Verification items for the finished model (mm, model axes). A direction names the side the tool comes from. Coordinates: 2 decimals unless noted, no trailing zeros. Order: outer loops, then holes, each group sorted by start corner. A loop starts at its lowest first (then second) coordinate and runs counter-clockwise, first axis right, second up. Notation, with made-up numbers: (-14.5, 8) -> (4.5, 8) arc R15 ccw to (4.5, 27) -> close; hole circle Ø5 at (45.25, -14). An arc over 180 degrees is marked (long way). Use CSV: the item, a comma, the result in double quotes. Start each with the question number.
1) Scan lines: line 1 along Z through (x, y) = (-4.25, -8); line 2 along X through (y, z) = (-0.5, 37); line 3 along X through (y, z) = (-4.25, 6.5). Record each from-to range of solid material in increasing order.
2) Sectioned sample at B-B on z = 7. Record the boundary of the cut face in (x, y).
3) Sectioned sample at D-D on y = 8.5. Record the boundary of the cut face in (x, z).
4) Tool access check on faces 1 (the flat face through (0, 7, 55)), 2 (the cylindrical face through (9.237, -3.83, 27.115)). Record the directions out of +Z, -Z, +X, -X, +Y, -Y that give a thin tool (end or side, any length) a straight path to the whole face; none if there is none.
5) Sectioned sample at A-A on y = -5.75. Record the boundary of the cut face in (x, z).
6) Go/stop test with flat-tipped pins: pin 1 (1 mm diameter, centred on x = -1.5, z = 12, fed in from -Y); pin 2 (6 mm diameter, centred on x = -6, z = 38.5, fed in from +Y); pin 3 (6 mm diameter, centred on x = -7, z = 16.5, fed in from -Y). Record where each tip stops, or that it passes through.
7) Sectioned sample at C-C on y = 3. Record the boundary of the cut face in (x, z), then the cut area to 3 significant figures.
8) Release check for a two-part mould opening along Y. For faces 3 (the flat face through (0, 5, 57)), 4 (the cylindrical face through (-0.14, 0.18, 3.29)), 5 (the flat face through (0, 0, 0)), 6 (the cylindrical face through (0, -7, 57)) record: released by +Y, released by -Y, zero draft, split by the parting line, or undercut.
from build123d import *

# Parameters (mm, degrees)
ESBO_O1_R                         = 10
RESSALTO_EXTRUS_O1_DEPTH          = 60
CORTE_EXTRUS_O1_START             = -5
ESBO_O7_R                         = 10
ESBO_O7_R_2                       = 7
CORTE_EXTRUS_O1_DEPTH             = 5
CORTE_EXTRUS_O2_START             = -5
CORTE_EXTRUS_O2_DEPTH             = 5
FURO_COM_FOLGA_DE_M21_D           = 2.6
FURO_COM_FOLGA_DE_M21_CSINK_D     = 2.65
FURO_COM_FOLGA_DE_M21_CSINK_ANGLE = 90


with BuildPart() as part:
    # Esboço1 → Ressalto-extrusão1 (new body)
    with BuildSketch(Plane.XY):
        Circle(ESBO_O1_R)
    extrude(amount=RESSALTO_EXTRUS_O1_DEPTH)

    # Esboço7 → Corte-extrusão1 (cut)
    with BuildSketch(Plane.XY.offset(60).offset(CORTE_EXTRUS_O1_START)):
        Circle(ESBO_O7_R)
        Circle(ESBO_O7_R_2, mode=Mode.SUBTRACT)
    extrude(amount=CORTE_EXTRUS_O1_DEPTH, mode=Mode.SUBTRACT)

    # Esboço9 → Corte-extrusão2 (cut)
    with BuildSketch(Plane.XY.offset(60).offset(CORTE_EXTRUS_O2_START)):
        with BuildLine():
            Line((-4.898979486, 5), (4.898979486, 5))
            ThreePointArc((4.898979486, 5), (0, 7), (-4.898979486, 5))
        make_face()
    extrude(amount=CORTE_EXTRUS_O2_DEPTH, mode=Mode.SUBTRACT)

    # Furo com folga de M21 (through all)
    with Locations(Plane(origin=(9.984543834, -0.555773718, 2), x_dir=(0.055577371817, 0.998454383406, 0), z_dir=(0.998454383406, -0.055577371817, 0))):
        with Locations((0, 0)):
            CounterSinkHole(FURO_COM_FOLGA_DE_M21_D / 2, FURO_COM_FOLGA_DE_M21_CSINK_D / 2, counter_sink_angle=FURO_COM_FOLGA_DE_M21_CSINK_ANGLE)


solid = part.part
Answers follow:
1,line 1,"z = 0 to 55"
1,line 2,"x = -9.99 to 9.99"
1,line 3,"x = -9.05 to 9.05"
2,outline,"circle Ø20 at (0, 0)"
3,outline,"(-5.27, 0) -> (5.27, 0) -> (5.27, 55) -> (-5.27, 55) -> close"
4,face 1,"+Z"
4,face 2,"+Z, -Z"
5,outline,"(-8.18, 0) -> (8.18, 0) -> (8.18, 55) -> (3.99, 55) -> (3.99, 60) -> (-3.99, 60) -> (-3.99, 55) -> (-8.18, 55) -> close"
6,pin 1,"stops at y = -9.95"
6,pin 2,"stops at y = 9.54"
6,pin 3,"stops at y = -9.17"
7,outline,"(-9.54, 0) -> (9.54, 0) -> (9.54, 55) -> (6.32, 55) -> (6.32, 60) -> (-6.32, 60) -> (-6.32, 55) -> (-9.54, 55) -> close"
7,area,"1,110 mm²"
8,face 3,"released by +Y"
8,face 4,"undercut"
8,face 5,"zero draft"
8,face 6,"split by the parting line"
